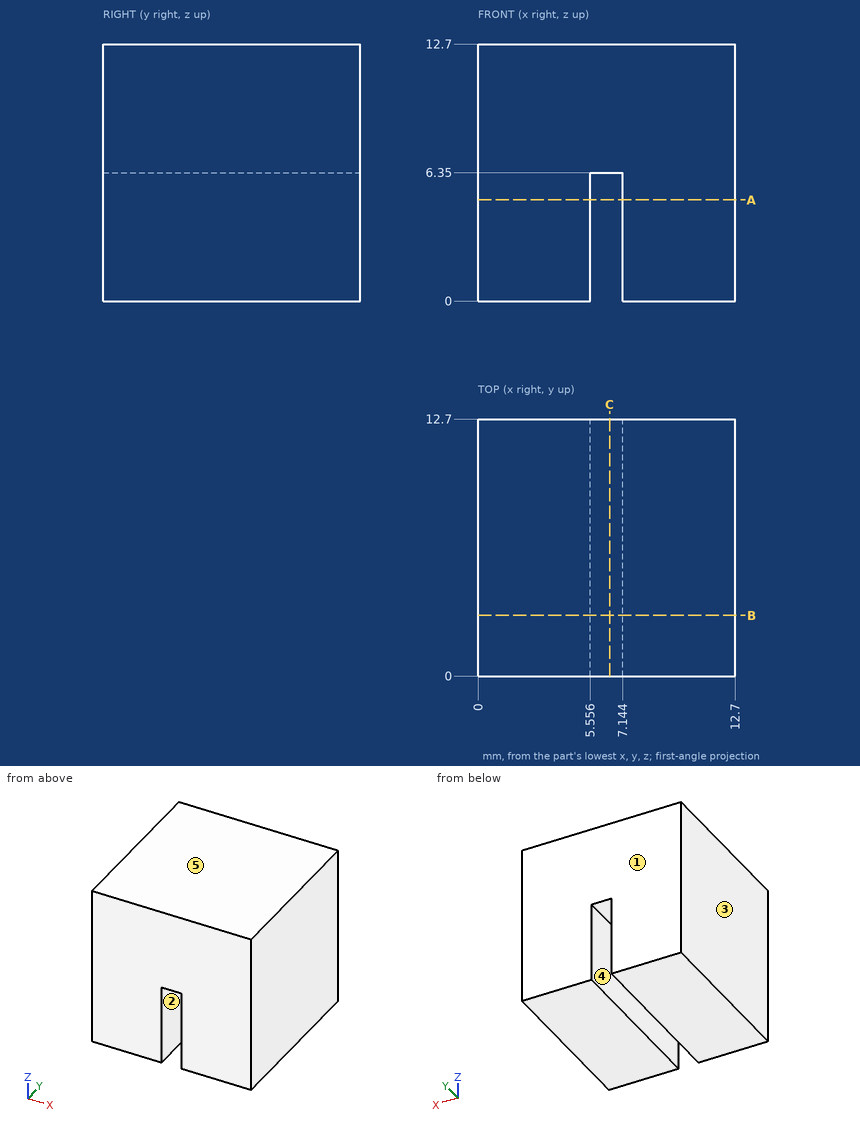
Verification items for this drawing (mm, ordinates from the low corner). A direction names the side the tool comes from. Give positions to 0.01 mm unless a question says otherwise; leave off trailing zeros. Write each loop counter-clockwise with the first axis right and the second up, starting at its lowest first coordinate (ties: lowest second). Pieces come first, ordered by that corner, then holes.
1) Release check for a two-part mould opening along X. For the marked faces 1, 2 and 3 record: released by +X, released by -X, zero draft, split by the parting line, or undercut.
Values follow:
face 1: zero draft
face 2: undercut
face 3: released by -X
2) Cross-section at A-A (z = 5). Record the boundary of the cut face in (x, y), plus the area to 3 significant figures.
Values follow:
outline: (0, 0) - (5.56, 0) - (5.56, 12.7) - (0, 12.7) - close; (7.14, 0) - (12.7, 0) - (12.7, 12.7) - (7.14, 12.7) - close
area: 141 mm2
3) Set-up check for the marked faces 4 and 5: record each of +Z, -Z, +X, -X, +Y, -Y from which the full face is reachable in a straight line by a thin tool's end or side.
Values follow:
face 4: -Z, +Y, -Y
face 5: +Z, +X, -X, +Y, -Y
4) Thickness scan on line 1 (X direction, y = 9.5, z = 5.75); line 2 (Z direction, x = 7, y = 8). Record the ranges inside material, lowest first.
Values follow:
line 1: x = 0 to 5.56, 7.14 to 12.7
line 2: z = 6.35 to 12.7
5) Go/stop test with a flat-tipped pin: pin 1 Ø0.8 at (x, y) = (6.5, 5) entering from -Z. Record where the tip stops, or that it passes through.
Values follow:
pin 1: stops at z = 6.35
6) Cross-section at B-B (y = 3). Record the boundary of the cut face in (x, z), plus the area to 3 significant figures.
Values follow:
outline: (0, 0) - (5.56, 0) - (5.56, 6.35) - (7.14, 6.35) - (7.14, 0) - (12.7, 0) - (12.7, 12.7) - (0, 12.7) - close
area: 151 mm2
7) Cross-section at C-C (x = 6.5). Record the boundary of the cut face in (y, z).
Values follow:
outline: (0, 6.35) - (12.7, 6.35) - (12.7, 12.7) - (0, 12.7) - close
